from build123d import *

# Parameters (mm, degrees)
SKETCH1_W                 = 12.22
SKETCH1_H                 = 11.1
BOSS_EXTRUDE1_DEPTH       = 9.65
SKETCH2_W                 = 5.78
SKETCH2_H                 = 0.7
CUT_EXTRUDE1_DEPTH        = 17.530378096
SKETCH4_W                 = 1.86
SKETCH4_H                 = 0.9
SKETCH4_W_2               = 1.16
CUT_EXTRUDE3_DEPTH        = 17.530378096
SKETCH5_W                 = 10.98
SKETCH5_H                 = 7.18
CUT_EXTRUDE4_DEPTH        = 0.9
SKETCH6_W                 = 3.37
SKETCH6_H                 = 7.18
BOSS_EXTRUDE2_DEPTH       = 7.45
SKETCH7_W                 = 0.8
SKETCH7_H                 = 1.27
BOSS_EXTRUDE3_DEPTH       = 2.25
SKETCH8_R                 = 0.601040764
CUT_EXTRUDE5_DEPTH        = 6.55
FILLET1_R                 = 0.2
SKETCH9_R                 = 1.375
CUT_EXTRUDE6_DEPTH        = 1.86
SKETCH11_W                = 3.37
SKETCH11_H                = 3.58
CUT_EXTRUDE8_DEPTH        = 2
CUT_EXTRUDE8_DRAFT        = -12
SKETCH12_R                = 0.815
CUT_EXTRUDE9_DEPTH        = 4.8
LPATTERN1_COUNT           = 3
LPATTERN1_PITCH           = 3.81
LPATTERN1_COPY_1_SKETCH_W = 3.37
LPATTERN1_COPY_1_SKETCH_H = 3.58
LPATTERN1_COPY_1_DEPTH    = 2
LPATTERN1_COPY_1_DRAFT    = -12
LPATTERN1_COPY_2_SKETCH_W = 3.37
LPATTERN1_COPY_2_SKETCH_H = 3.58
LPATTERN1_COPY_2_DEPTH    = 2
LPATTERN1_COPY_2_DRAFT    = -12
FILLET1_OF_LPATTERN1_R    = 0.2
SKETCH10_W                = 0.44
SKETCH10_H                = 1.555090365
CUT_EXTRUDE7_DEPTH        = 1.86
LPATTERN2_COUNT           = 2
LPATTERN2_PITCH           = 3.81


with BuildPart() as part:
    # Sketch1 → Boss-Extrude1 (new body)
    with BuildSketch(Plane(origin=(0, 0, 0), x_dir=(1, 0, 0), z_dir=(0, 1, 0))):
        Rectangle(SKETCH1_W, SKETCH1_H)
    extrude(amount=BOSS_EXTRUDE1_DEPTH)

    # Sketch2 → Cut-Extrude1 (cut, through all)
    with BuildSketch(Plane(origin=(6.11, 0, 0), x_dir=(0, 0, -1), z_dir=(1, 0, 0))):
        Polygon((-1.23, 9.65), (-1.23, 8.35), (-5.25, 7.6), (-5.25, 7.7), (-5.55, 7.7), (-5.55, 9.65), align=None)
        with Locations((2.66, 9.3)):
            Rectangle(SKETCH2_W, SKETCH2_H)
    extrude(amount=-CUT_EXTRUDE1_DEPTH, mode=Mode.SUBTRACT)

    # Sketch4 → Cut-Extrude3 (cut, through all)
    with BuildSketch(Plane(origin=(6.11, 0, 0), x_dir=(0, 0, -1), z_dir=(1, 0, 0))):
        with Locations((-4.62, 0.45)):
            Rectangle(SKETCH4_W, SKETCH4_H)
        with Locations((4.97, 0.45)):
            Rectangle(SKETCH4_W_2, SKETCH4_H)
    extrude(amount=-CUT_EXTRUDE3_DEPTH, mode=Mode.SUBTRACT)

    # Sketch5 → Cut-Extrude4 (cut)
    with BuildSketch(Plane.XZ):
        with Locations((0, -0.8)):
            Rectangle(SKETCH5_W, SKETCH5_H)
    extrude(amount=-CUT_EXTRUDE4_DEPTH, mode=Mode.SUBTRACT)

    # Sketch6 → Boss-Extrude2 (add)
    with BuildSketch(Plane.XZ.offset(-0.9)):
        with Locations((3.805, -0.8)):
            Rectangle(SKETCH6_W, SKETCH6_H)
    boss_extrude2 = extrude(amount=BOSS_EXTRUDE2_DEPTH)

    # Sketch7 → Boss-Extrude3 (add)
    with BuildSketch(Plane.XZ.offset(6.55)):
        with Locations((3.805, 3.425)):
            Rectangle(SKETCH7_W, SKETCH7_H)
    boss_extrude3 = extrude(amount=-BOSS_EXTRUDE3_DEPTH)

    # Sketch8 → Cut-Extrude5 (cut)
    with BuildSketch(Plane.XZ.offset(6.55)):
        with Locations(Location((3.805, 0.545, 0), (0, 0, 270))):
            Circle(SKETCH8_R)
        with BuildLine():
            Line((2.12, -1.7), (2.905, -1.7))
            ThreePointArc((2.905, -1.7), (3.805, -1.34), (4.705, -1.7))
            Line((4.705, -1.7), (5.49, -1.7))
            Line((5.49, -1.7), (5.49, -4.39))
            Line((5.49, -4.39), (2.12, -4.39))
            Line((2.12, -4.39), (2.12, -1.7))
        make_face()
    cut_extrude5 = extrude(amount=-CUT_EXTRUDE5_DEPTH, mode=Mode.SUBTRACT)

    # Fillet1
    fillet1_edges = [part.edges().sort_by_distance(p)[0] for p in [
        (3.805, -6.55, 1.146040764),
    ]]
    fillet(fillet1_edges, radius=FILLET1_R)

    # Sketch9 → Cut-Extrude6 (cut)
    with BuildSketch(Plane.XY.offset(5.55)):
        with Locations((3.805, 3.7)):
            Circle(SKETCH9_R)
        with BuildLine():
            Line((2.12, 2.455090365), (2.12, 0.9))
            Line((2.12, 0.9), (5.49, 0.9))
            Line((5.49, 0.9), (5.49, 2.455090365))
            ThreePointArc((5.49, 2.455090365), (3.805, 1.605), (2.12, 2.455090365))
        make_face()
    cut_extrude6 = extrude(amount=-CUT_EXTRUDE6_DEPTH, mode=Mode.SUBTRACT)


with BuildPart() as cut_extrude8_tool:
    # Sketch11 → Cut-Extrude8 (with draft: the straight prism first)
    with BuildSketch(Plane(origin=(0, 8.95, 0), x_dir=(1, 0, 0), z_dir=(0, 1, 0))):
        with Locations((3.805, 2.56)):
            Rectangle(SKETCH11_W, SKETCH11_H)
    extrude(amount=-CUT_EXTRUDE8_DEPTH)
    # Cut-Extrude8: the draft: its side faces are tilted about the plane it starts from
    cut_extrude8_sides = [cut_extrude8_tool.faces().sort_by_distance(p)[0] for p in [
        (5.49, 7.95, -2.56),
        (3.805, 7.95, -4.35),
        (2.12, 7.95, -2.56),
        (3.805, 7.95, -0.77),
    ]]
    draft(cut_extrude8_sides, Plane(origin=(0, 8.95, 0), x_dir=(1, 0, 0), z_dir=(0, 1, 0)), CUT_EXTRUDE8_DRAFT)


with BuildPart() as part_1:
    add(part.part)

    # Cut-Extrude8: cut by cut_extrude8_tool
    add(cut_extrude8_tool.part, mode=Mode.SUBTRACT)

    # Sketch12 → Cut-Extrude9 (cut)
    with BuildSketch(Plane(origin=(0, 6.95, 0), x_dir=(1, 0, 0), z_dir=(0, 1, 0))):
        with Locations(Location((3.805, 2.56, 0), (0, 0, 270))):
            Circle(SKETCH12_R)
    cut_extrude9 = extrude(amount=-CUT_EXTRUDE9_DEPTH, mode=Mode.SUBTRACT)

    # LPattern1: Boss-Extrude2, Boss-Extrude3, Cut-Extrude5, Cut-Extrude6, Cut-Extrude9 ×3
    with Locations(*[(-i * LPATTERN1_PITCH, 0, 0) for i in range(1, LPATTERN1_COUNT)]):
        add(boss_extrude2)
        add(boss_extrude3)
        add(cut_extrude5, mode=Mode.SUBTRACT)
        add(cut_extrude6, mode=Mode.SUBTRACT)
        add(cut_extrude9, mode=Mode.SUBTRACT)


with BuildPart() as lpattern1_copy_1_tool:
    # LPattern1 copy 1 sketch → LPattern1 copy 1 (with draft: the straight prism first)
    with BuildSketch(Plane(origin=(-3.81, 8.95, 0), x_dir=(1, 0, 0), z_dir=(0, 1, 0))):
        with Locations((3.805, 2.56)):
            Rectangle(LPATTERN1_COPY_1_SKETCH_W, LPATTERN1_COPY_1_SKETCH_H)
    extrude(amount=-LPATTERN1_COPY_1_DEPTH)
    # LPattern1 copy 1: the draft: its side faces are tilted about the plane it starts from
    lpattern1_copy_1_sides = [lpattern1_copy_1_tool.faces().sort_by_distance(p)[0] for p in [
        (1.68, 7.95, -2.56),
        (-0.005, 7.95, -4.35),
        (-1.69, 7.95, -2.56),
        (-0.005, 7.95, -0.77),
    ]]
    draft(lpattern1_copy_1_sides, Plane(origin=(-3.81, 8.95, 0), x_dir=(1, 0, 0), z_dir=(0, 1, 0)), LPATTERN1_COPY_1_DRAFT)


with BuildPart() as part_2:
    add(part_1.part)

    # LPattern1 copy 1: cut by lpattern1_copy_1_tool
    add(lpattern1_copy_1_tool.part, mode=Mode.SUBTRACT)


with BuildPart() as lpattern1_copy_2_tool:
    # LPattern1 copy 2 sketch → LPattern1 copy 2 (with draft: the straight prism first)
    with BuildSketch(Plane(origin=(-7.62, 8.95, 0), x_dir=(1, 0, 0), z_dir=(0, 1, 0))):
        with Locations((3.805, 2.56)):
            Rectangle(LPATTERN1_COPY_2_SKETCH_W, LPATTERN1_COPY_2_SKETCH_H)
    extrude(amount=-LPATTERN1_COPY_2_DEPTH)
    # LPattern1 copy 2: the draft: its side faces are tilted about the plane it starts from
    lpattern1_copy_2_sides = [lpattern1_copy_2_tool.faces().sort_by_distance(p)[0] for p in [
        (-2.13, 7.95, -2.56),
        (-3.815, 7.95, -4.35),
        (-5.5, 7.95, -2.56),
        (-3.815, 7.95, -0.77),
    ]]
    draft(lpattern1_copy_2_sides, Plane(origin=(-7.62, 8.95, 0), x_dir=(1, 0, 0), z_dir=(0, 1, 0)), LPATTERN1_COPY_2_DRAFT)


with BuildPart() as part_3:
    add(part_2.part)

    # LPattern1 copy 2: cut by lpattern1_copy_2_tool
    add(lpattern1_copy_2_tool.part, mode=Mode.SUBTRACT)

    # Fillet1 of LPattern1
    fillet1_of_lpattern1_edges = [part_3.edges().sort_by_distance(p)[0] for p in [
        (-0.005, -6.55, 1.146040764),
        (-3.815, -6.55, 1.146040764),
    ]]
    fillet(fillet1_of_lpattern1_edges, radius=FILLET1_OF_LPATTERN1_R)

    # Sketch10 → Cut-Extrude7 (cut)
    with BuildSketch(Plane.XY.offset(5.55)):
        with Locations((1.9, 1.677545183)):
            Rectangle(SKETCH10_W, SKETCH10_H)
    cut_extrude7 = extrude(amount=-CUT_EXTRUDE7_DEPTH, mode=Mode.SUBTRACT)

    # LPattern2: Cut-Extrude7 ×2
    with Locations(*[(-i * LPATTERN2_PITCH, 0, 0) for i in range(1, LPATTERN2_COUNT)]):
        add(cut_extrude7, mode=Mode.SUBTRACT)


solid = part_3.part
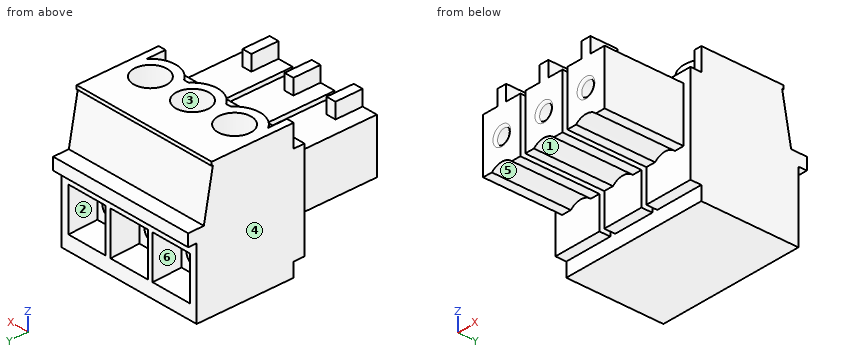
Design review of the part built by this model. Coordinates are the model's own, in mm. Face numbers are marked on the shaded views. A direction names the side the tool comes from. Give positions to 0.01 mm unless a question says otherwise; leave off trailing zeros. Loops run counter-clockwise (first coordinate to the right, second up) from the corner with the lowest first, then second, coordinate; pieces in that order, holes last. Notation, with made-up numbers: (58, 82) - (101, 82) arc R28 cw to (101, 117) - close; hole circle Ø8 at (1, 13.25). An arc over 180 degrees is marked (long way). Use CSV: the item, a comma, the result in double quotes. Start each with the question number.
1. Add section D-D (y = 3.7). State the section outline as (x, z) points (3 decimals).
2. Machinability: for the marked faces 1, 2 and 3, which of the approach directions +Z, -Z, +X, -X, +Y, -Y give a long, thin tool a straight path to every point of the face, cutting with its end or side? Answer none if there is none.
3. Insertion check: P1, Ø1, axis at x = 3.5, y = -2, coming from the +Z side; P2, Ø2, axis at x = 2, y = 1, coming from the +Z side; P3, Ø0.6, axis at x = -4, y = -5, coming from the +Z side. Each pin has a flat end and moves straight along its axis. Give the tip position at first contact, or say it passes through.
4. Wall thickness on L1, parallel to Y at x = 0, z = -3.75; L2, parallel to X at y = 3.25, z = -2; L3, parallel to Z at x = 0, y = 3.75: over which ranges is each line inside the solid? List them lowest first.
5. Add section B-B (y = -1.5). State the section outline as (x, z) points (3 decimals), plus the area to 3 significant figures.
6. Draft analysis for pull direction Z (two halves, no side actions). For the marked faces 4, 5 and 6, state which applies: released by +Z, released by -Z, zero draft, split by the parting line, or undercut.
7. Add section A-A (y = -4.5). Count the separate pieces of the cut face and the enclosed holes in it, plus the area to 3 significant figures.
8. Add section C-C (z = 2.5). State the section outline as (x, y) points.
Results found:
1,outline,"(-6.11, -5.55) - (6.11, -5.55) - (6.11, 5.55) - (5.18, 5.55) - (5.18, 3.69) - (2.43, 3.69) - (2.43, 5.55) - (1.37, 5.55) - (1.37, 3.69) - (-1.38, 3.69) - (-1.38, 5.55) - (-2.44, 5.55) - (-2.44, 3.69) - (-5.19, 3.69) - (-5.19, 5.55) - (-6.11, 5.55) - close; hole circle Ø1.63 at (-3.815, -2.56); hole circle Ø1.63 at (-0.005, -2.56); hole circle Ø1.63 at (3.805, -2.56)"
2,face 1,"-Z, -Y"
2,face 2,"+Y"
2,face 3,"+Z"
3,P1,"stops at z = 2.79"
3,P2,"stops at z = 3.69"
3,P3,"stops at z = 4.06"
4,L1,"y = 0 to 6.95"
4,L2,"x = -6.11 to -4.41, -3.22 to -0.6, 0.59 to 3.21, 4.4 to 6.11"
4,L3,"z = -5.55 to -3.37, -1.75 to 3.69"
5,outline,"(-5.5, -1.7) - (-4.715, -1.7) arc R1.305 cw to (-2.915, -1.7) - (-2.13, -1.7) - (-2.13, 2.79) - (-5.5, 2.79) - close; (-1.69, -1.7) - (-0.905, -1.7) arc R1.305 cw to (0.895, -1.7) - (1.68, -1.7) - (1.68, 2.79) - (-1.69, 2.79) - close; (2.12, -1.7) - (2.905, -1.7) arc R1.305 cw to (4.705, -1.7) - (5.49, -1.7) - (5.49, 2.79) - (2.12, 2.79) - close; hole circle Ø1.202 at (-3.815, 0.545); hole circle Ø1.202 at (-0.005, 0.545); hole circle Ø1.202 at (3.805, 0.545)"
5,area,"40.7 mm²"
6,face 4,"zero draft"
6,face 5,"released by -Z"
6,face 6,"undercut"
7,separate pieces,"3"
7,enclosed holes,"3"
7,area,"43.7 mm²"
8,outline,"(-6.11, 0) - (-5.5, 0) - (-5.5, -6.55) - (-2.13, -6.55) - (-2.13, 0.9) - (-1.69, 0.9) - (-1.69, -6.55) - (1.68, -6.55) - (1.68, 0.9) - (2.12, 0.9) - (2.12, -6.55) - (5.49, -6.55) - (5.49, 0) - (6.11, 0) - (6.11, 8.11) - (-6.11, 8.11) - close"
